For this review, take the finished solid that the model builds, in its own axes (mm). A direction names the side the tool comes from. Give positions to 0.01 mm unless a question says otherwise; leave off trailing zeros. Order: outer loops, then holes, each group sorted by start corner. A loop starts at its lowest first (then second) coordinate and runs counter-clockwise, first axis right, second up. Notation, with made-up numbers: (-16.75, -31) - (22.25, -31) arc R26 cw to (22.25, -8) - close; hole circle Ø2 at (56, 61). An arc over 180 degrees is marked (long way). One line per item, written item: value.
```python
from build123d import *

# Parameters (mm, degrees)
BOSS_EXTRUDE1_DEPTH = 5
SKETCH4_R           = 2
CUT_EXTRUDE1_DEPTH  = 6
SKETCH5_R           = 1
CUT_EXTRUDE2_DEPTH  = 3


with BuildPart() as part:
    # Sketch1 → Boss-Extrude1 (new body)
    with BuildSketch(Plane.XY):
        with BuildLine():
            Line((0, -43.5), (0, 43.5))
            ThreePointArc((0, 43.5), (1.464466094, 47.035533906), (5, 48.5))
            Line((5, 48.5), (87.5, 48.5))
            ThreePointArc((87.5, 48.5), (89.267766953, 47.767766953), (90, 46))
            Line((90, 46), (90, 43))
            ThreePointArc((90, 43), (89.267766953, 41.232233047), (87.5, 40.5))
            Line((87.5, 40.5), (10.5, 40.5))
            ThreePointArc((10.5, 40.5), (8.732233047, 39.767766953), (8, 38))
            Line((8, 38), (8, -38))
            ThreePointArc((8, -38), (8.732233047, -39.767766953), (10.5, -40.5))
            Line((10.5, -40.5), (87.5, -40.5))
            ThreePointArc((87.5, -40.5), (89.267766953, -41.232233047), (90, -43))
            Line((90, -43), (90, -46))
            ThreePointArc((90, -46), (89.267766953, -47.767766953), (87.5, -48.5))
            Line((87.5, -48.5), (5, -48.5))
            ThreePointArc((5, -48.5), (1.464466094, -47.035533906), (0, -43.5))
        make_face()
    extrude(amount=BOSS_EXTRUDE1_DEPTH)

    # Sketch4 → Cut-Extrude1 (cut, through all)
    with BuildSketch(Plane.XY.offset(5)):
        with Locations((71, 44.5)):
            Circle(SKETCH4_R)
        with Locations((31, 44.5)):
            Circle(SKETCH4_R)
        with Locations((71, -44.5)):
            Circle(SKETCH4_R)
        with Locations((31, -44.5)):
            Circle(SKETCH4_R)
        with Locations((51, 44.5)):
            Circle(SKETCH4_R)
    extrude(amount=-CUT_EXTRUDE1_DEPTH, mode=Mode.SUBTRACT)

    # Sketch5 → Cut-Extrude2 (cut)
    with BuildSketch(Plane.XY.offset(5)):
        with Locations((4, 44.5)):
            Circle(SKETCH5_R)
        with Locations((4, 0)):
            Circle(SKETCH5_R)
        with Locations((4, -44.5)):
            Circle(SKETCH5_R)
    extrude(amount=-CUT_EXTRUDE2_DEPTH, mode=Mode.SUBTRACT)


solid = part.part
```
(1) For P1, Ø3, axis at y = -31, z = 2, coming from the +X side; P2, Ø1, axis at x = 4.5, y = -44, coming from the +Z side; P3, Ø1.2, axis at x = 4, y = 44.5, coming from the +Z side, all flat-tipped, find the tip position at first contact; note any pin that passes through.
Answers below:
P1: stops at x = 8
P2: stops at z = 5
P3: stops at z = 2
(2) Draft analysis for pull direction Y (two halves, no side actions). For faces 4 (the face through (89, 48, 2)), 5 (the face through (4, -44, 2)), 6 (the face through (90, 45, 2)), state which applies: pulls with the +Y half, pulls with the -Y half, needs draft (parallel to the pull), parting line crosses it, or undercut.
Answers below:
face 4: pulls with the +Y half
face 5: undercut
face 6: needs draft
(3) Take a section at A-A (x = 51). Write out the cut boundary in (y, z), then the cut area to 3 significant figures.
Answers below:
outline: (-48.5, 0) - (-40.5, 0) - (-40.5, 5) - (-48.5, 5) - close; (40.5, 0) - (42.5, 0) - (42.5, 5) - (40.5, 5) - close; (46.5, 0) - (48.5, 0) - (48.5, 5) - (46.5, 5) - close
area: 60.0 mm^2
(4) Wall thickness on line 1 (Y direction, x = 51, z = 3.65); line 2 (Y direction, x = 71, z = 3.7); line 3 (Y direction, x = 58, z = 1.6): over which ranges is each line inside the solid? List them lowest first. Write a range as from..to.
Answers below:
line 1: y = -48.5..-40.5, 40.5..42.5, 46.5..48.5
line 2: y = -48.5..-46.5, -42.5..-40.5, 40.5..42.5, 46.5..48.5
line 3: y = -48.5..-40.5, 40.5..48.5
(5) Take a section at C-C (z = 3.1). Give the number of separate pieces and of enclosed holes in the cut face, then the cut area to 3 significant figures.
Answers below:
separate pieces: 1
enclosed holes: 8
area: 2,000 mm^2
(6) Machinability: for faces 1 (the face through (31.923, -46.274, 2.535)), 2 (the face through (89, -41, 2)), 3 (the face through (3.87, -43.51, 3.52)), which of the approach directions +Z, -Z, +X, -X, +Y, -Y give a long, thin tool a straight path to every point of the face, cutting with its end or side? Answer none if there is none.
Answers below:
face 1: +Z, -Z
face 2: +Z, -Z, +X
face 3: +Z
(7) Take a section at D-D (x = 81.5). Write out the cut boundary in (y, z).
Answers below:
outline: (-48.5, 0) - (-40.5, 0) - (-40.5, 5) - (-48.5, 5) - close; (40.5, 0) - (48.5, 0) - (48.5, 5) - (40.5, 5) - close
(8) Take a section at B-B (x = 31). Write out the cut boundary in (y, z).
Answers below:
outline: (-48.5, 0) - (-46.5, 0) - (-46.5, 5) - (-48.5, 5) - close; (-42.5, 0) - (-40.5, 0) - (-40.5, 5) - (-42.5, 5) - close; (40.5, 0) - (42.5, 0) - (42.5, 5) - (40.5, 5) - close; (46.5, 0) - (48.5, 0) - (48.5, 5) - (46.5, 5) - close
